Build history of the part. All positions in model axes, mm. Face numbers are marked on the shaded views. A direction names the side the tool comes from. Round coordinates to 2 decimals unless told otherwise and drop trailing zeros. Order: outer loops, then holes, each group sorted by start corner. A loop starts at its lowest first (then second) coordinate and runs counter-clockwise, first axis right, second up. Notation, with made-up numbers: (-19, 23) -> (34, 23) arc R18 cw to (34, 48) -> close; hole circle Ø3 at (13.25, 80.5). An arc over 180 degrees is marked (long way). Use a Markdown table: item, result. Add a question column.
Item 1: Probe L1, parallel to Y at x = 9, z = 1.5; L2, parallel to Z at x = 5.25, y = 94.75; L3, parallel to X at y = 98.5, z = 2.5. List the from-to ranges inside material, lowest first.
Item 2: Slice it at B-B, the plane x = 9.5. Give the cut face in (y, z).
Item 3: Slice it at A-A, the plane y = 89.5. Give the cut face in (x, z), plus the area to 3 significant figures.
Item 4: Pin check, flat tips, straight feed: pin 1 (0.7 mm diameter, centred on x = -2, z = 1.5, fed in from -Y); pin 2 (6.5 mm diameter, centred on x = 8.5, y = 95.5, fed in from -Z); pin 3 (3 mm diameter, centred on y = 82.5, z = 0.5, fed in from -X). Stop position of each tip, or through.
Item 5: Slice it at C-C, the plane y = 79.25. Give the cut face in (x, z), plus the area to 3 significant figures.
Item 6: 3-axis set-ups, long thin cutter, end or side, ignore diameter. For the marked faces 1, 2 and 3: which of +Z, -Z, +X, -X, +Y, -Y reach the whole face in a straight line?
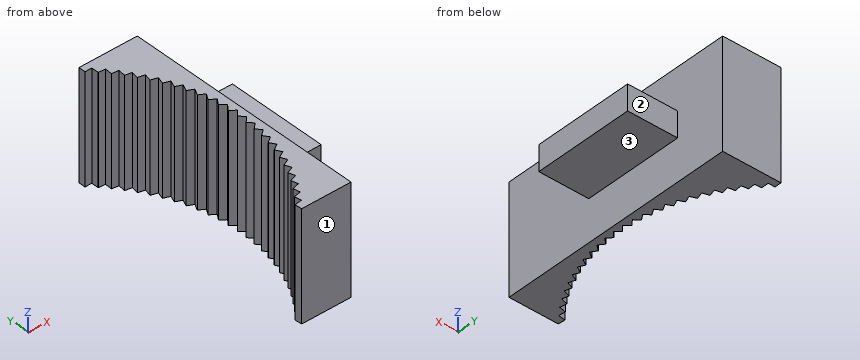
from build123d import *

# Parameters (mm, degrees)
SKETCH2_W           = 3.05
SKETCH2_H           = 11.9875
BOSS_EXTRUDE1_DEPTH = 6
SKETCH3_W           = 13.025
SKETCH3_H           = 28.832473971
BOSS_EXTRUDE2_DEPTH = 7
CUT_EXTRUDE1_DEPTH  = 108.108978223
CUT_EXTRUDE2_DEPTH  = 108.108978223
CUT_EXTRUDE5_DEPTH  = 108.108978223


with BuildPart() as part:
    # Sketch2 → Boss-Extrude1 (new body)
    with BuildSketch(Plane.ZY.offset(-4.42928947)):
        with Locations((1.625, 93.723397238)):
            Rectangle(SKETCH2_W, SKETCH2_H)
    extrude(amount=-BOSS_EXTRUDE1_DEPTH)

    # Sketch3 → Boss-Extrude2 (add)
    with BuildSketch(Plane.ZY.offset(-4.42928947)):
        with Locations((1.625, 91.385050871)):
            Rectangle(SKETCH3_W, SKETCH3_H)
    extrude(amount=BOSS_EXTRUDE2_DEPTH)

    # Sketch4 → Cut-Extrude1 (cut, through all)
    with BuildSketch(Plane(origin=(0, 0, -4.8875), x_dir=(-1, 0, 0), z_dir=(0, 0, -1))):
        with BuildLine():
            Line((2.304557749, 76.968813885), (2.57071053, 76.968813885))
            Line((2.57071053, 76.968813885), (2.57071053, 104.985183039))
            ThreePointArc((2.57071053, 104.985183039), (-3.287898054, 91.031390461), (2.304557749, 76.968813885))
        make_face()
    extrude(amount=-CUT_EXTRUDE1_DEPTH, mode=Mode.SUBTRACT)

    # Sketch5 → Cut-Extrude2 (cut, through all)
    with BuildSketch(Plane(origin=(0, 0, -4.8875), x_dir=(-1, 0, 0), z_dir=(0, 0, -1))):
        with BuildLine():
            Line((1.754605713, 104.985183039), (1.754605713, 104.119213356))
            ThreePointArc((1.754605713, 104.119213356), (2.156216431, 104.558268957), (2.57071053, 104.985183039))
            Line((2.57071053, 104.985183039), (1.754605713, 104.985183039))
        make_face()
        with BuildLine():
            Line((1.489258694, 76.983594993), (2.352806951, 76.918880997))
            ThreePointArc((2.352806951, 76.918880997), (1.944991444, 77.352179397), (1.550246284, 77.797417816))
            Line((1.550246284, 77.797417816), (1.489258694, 76.983594993))
        make_face()
        with BuildLine():
            Line((0.687749631, 77.91873396), (1.545882082, 77.802492021))
            ThreePointArc((1.545882082, 77.802492021), (1.164709557, 78.259403935), (0.797298045, 78.727452834))
            Line((0.797298045, 78.727452834), (0.687749631, 77.91873396))
        make_face()
        with BuildLine():
            Line((-0.056399641, 78.900132721), (0.793245114, 78.732778955))
            ThreePointArc((0.793245114, 78.732778955), (0.440080068, 79.211668756), (0.101317444, 79.700852644))
            Line((0.101317444, 79.700852644), (-0.056399641, 78.900132721))
        make_face()
        with BuildLine():
            Line((-0.74052526, 79.924278124), (0.097590291, 79.706411614))
            ThreePointArc((0.097590291, 79.706411614), (-0.226303036, 80.205565001), (-0.53520409, 80.714132724))
            Line((-0.53520409, 80.714132724), (-0.74052526, 79.924278124))
        make_face()
        with BuildLine():
            Line((-1.362178233, 80.987503993), (-0.538592123, 80.719904644))
            ThreePointArc((-0.538592123, 80.719904644), (-0.832054276, 81.237534778), (-1.109987975, 81.763665797))
            Line((-1.109987975, 81.763665797), (-1.362178233, 80.987503993))
        make_face()
        with BuildLine():
            Line((-1.919133205, 82.086004256), (-1.113024759, 81.769630004))
            ThreePointArc((-1.113024759, 81.769630004), (-1.375005221, 82.303883903), (-1.620976635, 82.845694806))
            Line((-1.620976635, 82.845694806), (-1.919133205, 82.086004256))
        make_face()
        with BuildLine():
            Line((-2.40939642, 83.215846566), (-1.623651299, 82.85182995))
            ThreePointArc((-1.623651299, 82.85182995), (-1.853212247, 83.400795124), (-2.066340861, 83.956346368))
            Line((-2.066340861, 83.956346368), (-2.40939642, 83.215846566))
        make_face()
        with BuildLine():
            Line((-2.831212865, 84.372986382), (-2.068643831, 83.962630487))
            ThreePointArc((-2.068643831, 83.962630487), (-2.264963498, 84.524341782), (-2.444486366, 85.091644638))
            Line((-2.444486366, 85.091644638), (-2.831212865, 84.372986382))
        make_face()
        with BuildLine():
            Line((-3.183072545, 85.553281444), (-2.446409398, 85.098055237))
            ThreePointArc((-2.446409398, 85.098055237), (-2.608785009, 85.670501873), (-2.754059488, 86.247525544))
            Line((-2.754059488, 86.247525544), (-3.183072545, 85.553281444))
        make_face()
        with BuildLine():
            Line((-3.463715894, 86.752506602), (-2.755595697, 86.254039674))
            ThreePointArc((-2.755595697, 86.254039674), (-2.88344599, 86.835172441), (-2.993952034, 87.419851331))
            Line((-2.993952034, 87.419851331), (-3.463715894, 86.752506602))
        make_face()
        with BuildLine():
            Line((-3.672138283, 87.96636894), (-2.995095921, 87.426445673))
            ThreePointArc((-2.995095921, 87.426445673), (-3.087963225, 88.014184267), (-3.163305252, 88.604425379))
            Line((-3.163305252, 88.604425379), (-3.672138283, 87.96636894))
        make_face()
        with BuildLine():
            Line((-3.807593612, 89.190523146), (-3.164052722, 88.611076327))
            ThreePointArc((-3.164052722, 88.611076327), (-3.221604597, 89.203316795), (-3.2615129, 89.797007218))
            Line((-3.2615129, 89.797007218), (-3.807593612, 89.190523146))
        make_face()
        with BuildLine():
            Line((-3.869596987, 90.420587067), (-3.261861279, 89.803690964))
            ThreePointArc((-3.261861279, 89.803690964), (-3.283891703, 90.39831324), (-3.288223422, 90.993327716))
            Line((-3.288223422, 90.993327716), (-3.869596987, 90.420587067))
        make_face()
        with BuildLine():
            Line((-3.857926452, 91.652157392), (-3.288171462, 91.000020333))
            ThreePointArc((-3.288171462, 91.000020333), (-3.274601572, 91.594895823), (-3.243341201, 92.189104356))
            Line((-3.243341201, 92.189104356), (-3.857926452, 91.652157392))
        make_face()
        with BuildLine():
            Line((-3.772623784, 92.88082542), (-3.242889087, 92.195781886))
            ThreePointArc((-3.242889087, 92.195781886), (-3.19376746, 92.788781091), (-3.127026902, 93.380056567))
            Line((-3.127026902, 93.380056567), (-3.772623784, 92.88082542))
        make_face()
        with BuildLine():
            Line((-3.613994345, 94.102192837), (-3.126176253, 93.386695107))
            ThreePointArc((-3.126176253, 93.386695107), (-3.041678732, 93.975695243), (-2.939696901, 94.56192105))
            Line((-2.939696901, 94.56192105), (-3.613994345, 94.102192837))
        make_face()
        with BuildLine():
            Line((-3.382605988, 95.311887466), (-2.938450763, 94.568496836))
            ThreePointArc((-2.938450763, 94.568496836), (-2.818879826, 95.151389435), (-2.682021792, 95.730467037))
            Line((-2.682021792, 95.730467037), (-3.382605988, 95.311887466))
        make_face()
        with BuildLine():
            Line((-3.079287021, 96.505578914), (-2.680384624, 95.736956529))
            ThreePointArc((-2.680384624, 95.736956529), (-2.526168306, 96.311654987), (-2.354923983, 96.881511437))
            Line((-2.354923983, 96.881511437), (-3.079287021, 96.505578914))
        make_face()
        with BuildLine():
            Line((-2.705123249, 97.678994074), (-2.352901647, 96.887891404))
            ThreePointArc((-2.352901647, 96.887891404), (-2.164592001, 97.45233845), (-1.959574401, 98.010933808))
            Line((-1.959574401, 98.010933808), (-2.705123249, 97.678994074))
        make_face()
        with BuildLine():
            Line((-2.261454081, 98.827932426), (-1.957174136, 98.017181412))
            ThreePointArc((-1.957174136, 98.017181412), (-1.735445261, 98.569356472), (-1.497388293, 99.114691113))
            Line((-1.497388293, 99.114691113), (-2.261454081, 98.827932426))
        make_face()
        with BuildLine():
            Line((-1.749867737, 99.948281069), (-1.494618692, 99.120783989))
            ThreePointArc((-1.494618692, 99.120783989), (-1.240264321, 99.658710419), (-0.970020167, 100.188832186))
            Line((-0.970020167, 100.188832186), (-1.749867737, 99.948281069))
        make_face()
        with BuildLine():
            Line((-1.172195564, 101.036029444), (-0.966891144, 100.194748523))
            ThreePointArc((-0.966891144, 100.194748523), (-0.680821799, 100.716500687), (-0.379357863, 101.229511882))
            Line((-0.379357863, 101.229511882), (-1.172195564, 101.036029444))
        make_face()
        with BuildLine():
            Line((-0.530505477, 102.087283695), (-0.375880619, 101.2352305))
            ThreePointArc((-0.375880619, 101.2352305), (-0.059120355, 101.738940661), (0.2724842, 102.233004837))
            Line((0.2724842, 102.233004837), (-0.530505477, 102.087283695))
        make_face()
        with BuildLine():
            Line((0.172905439, 103.098280604), (0.276297217, 102.238505266))
            ThreePointArc((0.276297217, 102.238505266), (0.622614482, 102.722370271), (0.983172598, 103.195718806))
            Line((0.983172598, 103.195718806), (0.172905439, 103.098280604))
        make_face()
        with BuildLine():
            Line((0.935519155, 104.065401066), (0.987307739, 103.200981356))
            ThreePointArc((0.987307739, 103.200981356), (1.361942278, 103.663269094), (1.75016325, 104.114207524))
            Line((1.75016325, 104.114207524), (0.935519155, 104.065401066))
        make_face()
    extrude(amount=-CUT_EXTRUDE2_DEPTH, mode=Mode.SUBTRACT)

    # Sketch6 → Cut-Extrude5 (cut, through all)
    with BuildSketch(Plane(origin=(0, 0, -4.8875), x_dir=(-1, 0, 0), z_dir=(0, 0, -1))):
        Polygon((1.489258694, 76.983594993), (1.488151003, 76.968813885), (1.686498876, 76.968813885), align=None)
    extrude(amount=-CUT_EXTRUDE5_DEPTH, mode=Mode.SUBTRACT)


solid = part.part
Check sheet entries:
| question | item | result |
|---|---|---|
| 1 | L1 | 87.73 to 99.72 |
| 1 | L2 | 0.1 to 3.15 |
| 1 | L3 | 2.14 to 10.43 |
| 2 | outline | (87.73, 0.1) -> (99.72, 0.1) -> (99.72, 3.15) -> (87.73, 3.15) -> close |
| 3 | outline | (3.53, -4.89) -> (4.43, -4.89) -> (4.43, 0.1) -> (10.43, 0.1) -> (10.43, 3.15) -> (4.43, 3.15) -> (4.43, 8.14) -> (3.53, 8.14) -> close |
| 3 | area | 30.0 mm2 |
| 4 | pin 1 | y = 104.11 |
| 4 | pin 2 | z = 0.1 |
| 4 | pin 3 | x = 1.11 |
| 5 | outline | (-0.01, -4.89) -> (4.43, -4.89) -> (4.43, 8.14) -> (-0.01, 8.14) -> close |
| 5 | area | 57.9 mm2 |
| 6 | face 1 | +Z, -Z, +X, -X, -Y |
| 6 | face 2 | +Z, -Z, +X, +Y |
| 6 | face 3 | -Z, +X, +Y, -Y |
